from build123d import *

# Parameters (mm, degrees)
SKETCH1_W           = 62
SKETCH1_H           = 42
BOSS_EXTRUDE1_DEPTH = 20
SKETCH8_W           = 24
SKETCH8_H           = 38
CUT_EXTRUDE1_DEPTH  = 11.5
CUT_EXTRUDE2_REACH  = 41.17
SKETCH9_R           = 8.5
SKETCH10_W          = 57
SKETCH10_H          = 23.165977038
CUT_EXTRUDE3_DEPTH  = 18
FILLET1_R           = 3
FILLET2_R           = 3
SKETCH11_W          = 18
SKETCH11_H          = 8
CUT_EXTRUDE4_DEPTH  = 8.5
SKETCH12_W          = 60
SKETCH12_H          = 40
CUT_EXTRUDE5_DEPTH  = 3
FILLET3_R           = 3
SKETCH13_W          = 18
SKETCH13_H          = 12
CUT_EXTRUDE6_DEPTH  = 7
CUT_EXTRUDE10_REACH = 44.45
SKETCH18_W          = 10.5
SKETCH18_H          = 7
SKETCH22_W          = 5
SKETCH22_H          = 14
BOSS_EXTRUDE2_DEPTH = 4
SKETCH16_R          = 2
CUT_EXTRUDE9_DEPTH  = 1.5
CHAMFER1_SIZE       = 1
SKETCH19_W          = 34
SKETCH19_H          = 1.2
CUT_EXTRUDE11_DEPTH = 16
SKETCH20_W          = 34
SKETCH20_H          = 0.717011481
CUT_EXTRUDE12_DEPTH = 10
SKETCH21_W          = 60
SKETCH21_H          = 8
CUT_EXTRUDE13_DEPTH = 10
SKETCH14_W          = 24.0014575
SKETCH14_H          = 44.120551562
CUT_EXTRUDE7_DEPTH  = 13
SKETCH15_W          = 25.642620831
SKETCH15_H          = 19.236744125
CUT_EXTRUDE8_DEPTH  = 10
SKETCH23_W          = 12
SKETCH23_H          = 0.717011481
CUT_EXTRUDE14_DEPTH = 5


with BuildPart() as part:
    # Sketch1 → Boss-Extrude1 (new body)
    with BuildSketch(Plane.XY):
        Rectangle(SKETCH1_W, SKETCH1_H)
    extrude(amount=BOSS_EXTRUDE1_DEPTH)

    # Sketch8 → Cut-Extrude1 (cut)
    with BuildSketch(Plane.XY.offset(20)):
        Rectangle(SKETCH8_W, SKETCH8_H)
    extrude(amount=-CUT_EXTRUDE1_DEPTH, mode=Mode.SUBTRACT)

    # Sketch9 → Cut-Extrude2 (cut, up to next)
    with BuildSketch(Plane.XY.offset(8.5), mode=Mode.PRIVATE) as cut_extrude2_sk1:
        with Locations((-0.494531145, 6)):
            Circle(SKETCH9_R)
    cut_extrude2_tool1 = extrude(cut_extrude2_sk1.sketch, amount=-CUT_EXTRUDE2_REACH, mode=Mode.PRIVATE) & part.part
    add(cut_extrude2_tool1.solids().sort_by_distance((-0.494531, 6, 8.5))[0], mode=Mode.SUBTRACT)

    # Sketch10 → Cut-Extrude3 (cut)
    with BuildSketch(Plane.XY.offset(20)):
        with Locations((0, 6)):
            Rectangle(SKETCH10_W, SKETCH10_H)
    extrude(amount=-CUT_EXTRUDE3_DEPTH, mode=Mode.SUBTRACT)

    # Fillet1
    fillet1_edges = [part.edges().sort_by_distance(p)[0] for p in [
        (-31, 0, 0),
        (0, -21, 0),
        (31, 0, 0),
        (0, 21, 0),
    ]]
    fillet(fillet1_edges, radius=FILLET1_R)

    # Fillet2
    # the kernel refuses this fillet: 3 mm, written as the material it takes off along each edge
    with BuildSketch(Plane(origin=(-28, 18, 3), x_dir=(-1, 0, 0), z_dir=(0, 1, 0))) as fillet2_piece_1_section:
        Polygon((0, 0), (FILLET2_R, 0), (FILLET2_R, -FILLET2_R), (0, -FILLET2_R), align=None)
    fillet2_piece_1 = extrude(amount=FILLET2_R, mode=Mode.PRIVATE)
    fillet2_piece_1 = fillet2_piece_1 - Plane(origin=(-28, 18, 3), x_dir=(0.7071067811865475, 0, 0.7071067811865475), z_dir=(0, 1, 0)) * Sphere(FILLET2_R, mode=Mode.PRIVATE)
    add(fillet2_piece_1, mode=Mode.SUBTRACT)
    with BuildSketch(Plane(origin=(-28, -18, 3), x_dir=(0, -1, 0), z_dir=(-1, 0, 0))) as fillet2_piece_2_section:
        Polygon((0, 0), (FILLET2_R, 0), (FILLET2_R, -FILLET2_R), (0, -FILLET2_R), align=None)
    fillet2_piece_2 = extrude(amount=FILLET2_R, mode=Mode.PRIVATE)
    fillet2_piece_2 = fillet2_piece_2 - Plane(origin=(-28, -18, 3), x_dir=(0, 0.7071067811865475, 0.7071067811865475), z_dir=(-1, 0, 0)) * Sphere(FILLET2_R, mode=Mode.PRIVATE)
    add(fillet2_piece_2, mode=Mode.SUBTRACT)
    with BuildSketch(Plane(origin=(28, 18, 3), x_dir=(1, 0, 0), z_dir=(0, 1, 0))) as fillet2_piece_3_section:
        Polygon((0, 0), (FILLET2_R, 0), (FILLET2_R, FILLET2_R), (0, FILLET2_R), align=None)
    fillet2_piece_3 = extrude(amount=FILLET2_R, mode=Mode.PRIVATE)
    fillet2_piece_3 = fillet2_piece_3 - Plane(origin=(28, 18, 3), x_dir=(-0.7071067811865475, 0, 0.7071067811865475), z_dir=(0, 1, 0)) * Sphere(FILLET2_R, mode=Mode.PRIVATE)
    add(fillet2_piece_3, mode=Mode.SUBTRACT)
    with BuildSketch(Plane(origin=(28, -18, 3), x_dir=(0, -1, 0), z_dir=(1, 0, 0))) as fillet2_piece_4_section:
        Polygon((0, 0), (FILLET2_R, 0), (FILLET2_R, FILLET2_R), (0, FILLET2_R), align=None)
    fillet2_piece_4 = extrude(amount=FILLET2_R, mode=Mode.PRIVATE)
    fillet2_piece_4 = fillet2_piece_4 - Plane(origin=(28, -18, 3), x_dir=(0, 0.7071067811865475, 0.7071067811865475), z_dir=(1, 0, 0)) * Sphere(FILLET2_R, mode=Mode.PRIVATE)
    add(fillet2_piece_4, mode=Mode.SUBTRACT)
    with BuildSketch(Plane(origin=(-31, 21, 3), x_dir=(1, 0, 0), z_dir=(0, 0, 1)), Plane(origin=(-31, -21, 3), x_dir=(0, 1, 0), z_dir=(0, 0, 1))) as fillet2_piece_5:
        with BuildLine():
            CenterArc((FILLET2_R, -FILLET2_R), FILLET2_R, 90, 90)
            Line((0, -FILLET2_R), (0, 0))
            Line((0, 0), (FILLET2_R, 0))
        make_face()
    extrude(amount=24.5, mode=Mode.SUBTRACT)
    with BuildSketch(Plane(origin=(31, -21, 3), x_dir=(0, 1, 0), z_dir=(0, 0, 1)), Plane(origin=(31, 21, 3), x_dir=(-1, 0, 0), z_dir=(0, 0, 1))) as fillet2_piece_6:
        with BuildLine():
            CenterArc((FILLET2_R, FILLET2_R), FILLET2_R, 180, 90)
            Line((0, FILLET2_R), (0, 0))
            Line((0, 0), (FILLET2_R, 0))
        make_face()
    extrude(amount=24.5, mode=Mode.SUBTRACT)

    # Sketch11 → Cut-Extrude4 (cut)
    with BuildSketch(Plane.XY.offset(20)):
        with Locations((0, -17)):
            Rectangle(SKETCH11_W, SKETCH11_H)
    extrude(amount=-CUT_EXTRUDE4_DEPTH, mode=Mode.SUBTRACT)

    # Sketch12 → Cut-Extrude5 (cut)
    with BuildSketch(Plane.XY.offset(20)):
        Rectangle(SKETCH12_W, SKETCH12_H)
    extrude(amount=-CUT_EXTRUDE5_DEPTH, mode=Mode.SUBTRACT)

    # Fillet3
    fillet3_edges = [part.edges().sort_by_distance(p)[0] for p in [
        (30, -20, 18.5),
        (-30, -20, 18.5),
        (-30, 20, 18.5),
        (30, 20, 18.5),
    ]]
    fillet(fillet3_edges, radius=FILLET3_R)

    # Sketch13 → Cut-Extrude6 (cut)
    with BuildSketch(Plane.XY.offset(8.5)):
        with Locations((0, -11.582988519)):
            Rectangle(SKETCH13_W, SKETCH13_H)
    extrude(amount=-CUT_EXTRUDE6_DEPTH, mode=Mode.SUBTRACT)

    # Sketch18 → Cut-Extrude10 (cut, up to next)
    with BuildSketch(Plane(origin=(0, 0, 0), x_dir=(-1, 0, 0), z_dir=(0, 0, -1)), mode=Mode.PRIVATE) as cut_extrude10_sk1:
        with Locations((-19.755468855, 6)):
            Rectangle(SKETCH18_W, SKETCH18_H)
    cut_extrude10_tool1 = extrude(cut_extrude10_sk1.sketch, amount=-CUT_EXTRUDE10_REACH, mode=Mode.PRIVATE) & part.part
    # Sketch18 → Cut-Extrude10 (cut, up to next)
    with BuildSketch(Plane(origin=(0, 0, 0), x_dir=(-1, 0, 0), z_dir=(0, 0, -1)), mode=Mode.PRIVATE) as cut_extrude10_sk2:
        with Locations((20.744531145, 6)):
            Rectangle(SKETCH18_W, SKETCH18_H)
    cut_extrude10_tool2 = extrude(cut_extrude10_sk2.sketch, amount=-CUT_EXTRUDE10_REACH, mode=Mode.PRIVATE) & part.part
    add(cut_extrude10_tool1.solids().sort_by_distance((19.755469, 6, 0))[0], mode=Mode.SUBTRACT)
    add(cut_extrude10_tool2.solids().sort_by_distance((-20.744531, 6, 0))[0], mode=Mode.SUBTRACT)

    # Sketch22 → Boss-Extrude2 (add)
    with BuildSketch(Plane.XY.offset(2)):
        with Locations((-11.994531145, 6)):
            Rectangle(SKETCH22_W, SKETCH22_H)
        with Locations((11.005468855, 6)):
            Rectangle(SKETCH22_W, SKETCH22_H)
    extrude(amount=BOSS_EXTRUDE2_DEPTH)

    # Sketch16 → Cut-Extrude9 (cut)
    with BuildSketch(Plane.XY.offset(6)):
        with Locations((-11.094531145, 6)):
            Circle(SKETCH16_R)
        with Locations((10.105468855, 6)):
            Circle(SKETCH16_R)
    extrude(amount=-CUT_EXTRUDE9_DEPTH, mode=Mode.SUBTRACT)

    # Chamfer1
    chamfer1_edges = [part.edges().sort_by_distance(p)[0] for p in [
        (25.005468855, 6, 0),
        (19.755468855, 2.5, 0),
        (14.505468855, 6, 0),
        (19.755468855, 9.5, 0),
        (-15.494531145, 6, 0),
        (-20.744531145, 2.5, 0),
        (-25.994531145, 6, 0),
        (-20.744531145, 9.5, 0),
    ]]
    chamfer(chamfer1_edges, length=CHAMFER1_SIZE)

    # Sketch19 → Cut-Extrude11 (cut)
    with BuildSketch(Plane.XY.offset(17)):
        with Locations((0.034121004, 18.9)):
            Rectangle(SKETCH19_W, SKETCH19_H)
    extrude(amount=-CUT_EXTRUDE11_DEPTH, mode=Mode.SUBTRACT)

    # Sketch20 → Cut-Extrude12 (cut)
    with BuildSketch(Plane.XY.offset(17)):
        with Locations((0.034121004, 17.94149426)):
            Rectangle(SKETCH20_W, SKETCH20_H)
    extrude(amount=-CUT_EXTRUDE12_DEPTH, mode=Mode.SUBTRACT)

    # Sketch21 → Cut-Extrude13 (cut)
    with BuildSketch(Plane.XY.offset(17)):
        with Locations((0, -9.582988519)):
            Rectangle(SKETCH21_W, SKETCH21_H)
    extrude(amount=-CUT_EXTRUDE13_DEPTH, mode=Mode.SUBTRACT)

    # Sketch14 → Cut-Extrude7 (cut)
    with BuildSketch(Plane.ZY.offset(31)):
        with Locations((10.285512598, -0.436155296)):
            Rectangle(SKETCH14_W, SKETCH14_H)
    extrude(amount=-CUT_EXTRUDE7_DEPTH, mode=Mode.SUBTRACT)

    # Sketch15 → Cut-Extrude8 (cut)
    with BuildSketch(Plane.ZY.offset(18)):
        with Locations((10.646983425, -12.09757059)):
            Rectangle(SKETCH15_W, SKETCH15_H)
    extrude(amount=-CUT_EXTRUDE8_DEPTH, mode=Mode.SUBTRACT)

    # Sketch23 → Cut-Extrude14 (cut)
    with BuildSketch(Plane.XY.offset(7)):
        with Locations((-10.965878996, 17.94149426)):
            Rectangle(SKETCH23_W, SKETCH23_H)
    extrude(amount=-CUT_EXTRUDE14_DEPTH, mode=Mode.SUBTRACT)


solid = part.part
Here's how the part is built. I have some questions about the finished solid (model axes, mm). A direction names the side the tool comes from. Give positions to 0.01 mm unless a question says otherwise; leave off trailing zeros. Loops run counter-clockwise (first coordinate to the right, second up) from the corner with the lowest first, then second, coordinate; pieces in that order, holes last. Notation, with made-up numbers: (88, 42) -> (134, 42) arc R33 cw to (134, 71) -> close; hole circle Ø2 at (20, -25.75). An arc over 180 degrees is marked (long way). One line per item, written item: value.
Q1. We'd pull the mould along Y, two halves only. Please class faces 1 (the face through (-8, -14, 1)), 2 (the face through (4, 18.3, 4)), 3 (the face through (14, -21, 9)): pulls with the +Y half, pulls with the -Y half, needs draft (parallel to the pull), parting line crosses it, or undercut.
Answers follow:
face 1: needs draft
face 2: undercut
face 3: pulls with the -Y half
Q2. Suppose I cut it at B-B on y = 6. State how many separate pieces and enclosed holes the cut face has, then the cut area to 3 significant figures.
Answers follow:
separate pieces: 3
enclosed holes: 0
area: 104 mm^2
Q3. Suppose I cut it at D-D on x = 15.5. Please give me the cut outline in (y, z), then the cut area to 3 significant figures.
Answers follow:
outline: (-21, 3) arc R3 ccw to (-18, 0) -> (1.5, 0) -> (2.5, 1) -> (2.5, 2) -> (-5.58, 2) -> (-5.58, 7) -> (-13.58, 7) -> (-13.58, 17) -> (-20, 17) -> (-20, 20) -> (-21, 20) -> close; (9.5, 1) -> (10.5, 0) -> (18, 0) arc R3 ccw to (21, 3) -> (21, 20) -> (20, 20) -> (20, 17) -> (19.5, 17) -> (19.5, 1) -> (18.3, 1) -> (18.3, 7) -> (17.58, 7) -> (17.58, 2) -> (9.5, 2) -> close
area: 247 mm^2
Q4. I'm going to push flat-ended pins straight in: pin 1 Ø2 at (y, z) = (-11.5, 15.5) entering from -X; pin 2 Ø6.5 at (y, z) = (-5, 11.5) entering from -X; pin 3 Ø5 at (y, z) = (4.5, 3) entering from -X; pin 4 Ø1 at (y, z) = (-20.5, 16) entering from -X. Where does each tip first touch, or does it pass through?
Answers follow:
pin 1: x = 30
pin 2: x = 28.5
pin 3: x = -18
pin 4: x = 9
Q5. On a 3-axis mill with a long thin cutter (end or side, diameter ignored), from which of +Z, -Z, +X, -X, +Y, -Y can I reach the whole of each face in a straight line? I mean faces 4 (the face through (-12, 13, 4)), 5 (the face through (10, 6, 4.5)), 6 (the face through (-18, 18, 8)), 7 (the face through (-17.5, 17.583, 9.6)). Say none if no direction works.
Answers follow:
face 4: +Z, -X
face 5: +Z
face 6: +Z, -Z, -X, +Y, -Y
face 7: +Z, -X, -Y
Q6. If I drill on line 1 along X through (y, z) = (6, 5.35); line 2 along Y through (x, z) = (4, 3.25); line 3 along X through (y, z) = (12.5, 3), over which ranges is the centre line in solid material (lowest first)?
Answers follow:
line 1: -14.49 to -13.09, 12.11 to 13.51, 28.5 to 31
line 2: -21 to -17.58, 17.58 to 18.3, 19.5 to 21
line 3: -14.49 to -9.49, 8.51 to 13.51, 28.5 to 31
Q7. Suppose I cut it at A-A on x = 23.5. Please give me the cut outline in (y, z).
Answers follow:
outline: (-21, 3) arc R3 ccw to (-18, 0) -> (1.5, 0) -> (2.5, 1) -> (2.5, 2) -> (-5.58, 2) -> (-5.58, 7) -> (-13.58, 7) -> (-13.58, 17) -> (-20, 17) -> (-20, 20) -> (-21, 20) -> close; (9.5, 1) -> (10.5, 0) -> (18, 0) arc R3 ccw to (21, 3) -> (21, 20) -> (20, 20) -> (20, 17) -> (17.58, 17) -> (17.58, 2) -> (9.5, 2) -> close
